Read the model definition and answer for the solid it produces. Units are mm, in the model's axes. Coordinates: 2 decimals unless noted, no trailing zeros. Order: outer loops, then holes, each group sorted by start corner. A loop starts at its lowest first (then second) coordinate and runs counter-clockwise, first axis right, second up. Notation, with made-up numbers: M 36.25,39.5 L 87.25,39.5 A29 cw 87.25,60.5 Z; hole C -4.75,-5.5 d4. An arc over 180 degrees is marked long. Use a Markdown table: item, result. Add a question column.
1) Find section C-C on y = -21.5. Write down the section's boundary in (x, z), plus the area to 3 significant figures.
2) Find section A-A on z = 1.6. Write down the section's boundary in (x, y).
3) Find the intervals of material crossed by probe 1 along Y at (x, z) = (126.5, 1.55); probe 2 along Y at (x, z) = (124.5, 1.7); probe 3 along X at (y, z) = (5.5, 0.7), in increasing order. Write a range as [from, to].
4) The mould has two halves that part along X. Classify faces 1 (the face through (159.386, 1.553, 1.972)), 2 (the face through (18, -14, 0)), 3 (the face through (-62.32, -15.34, 1.97)), 4 (the face through (139.64, -15, 1.97)): released by +X, released by -X, zero draft, split by the parting line, or undercut.
5) Find section B-B on x = 15.5. Write down the section's boundary in (y, z), plus the area to 3 significant figures.
from build123d import *

# Parameters (mm, degrees)
BOSS_EXTRUDE1_DEPTH = 4
FILLET1_R           = 2
FILLET2_R           = 6


with BuildPart() as part:
    # Sketch1 → Boss-Extrude1 (new body)
    with BuildSketch(Plane.XY):
        Polygon((0, 0), (145, 0), (148.090169944, -9.510565163), (157.125206849, -6.574903716), (152.040911292, 9.072949017), (154.894080841, 10), (166.551226371, -11.92390211), (147.252212567, -18.194531813), (132.5, -12), (0, -26.511110048), (-119.286760587, -39.57513503), (-122.91114097, -30.255056337), align=None)
    extrude(amount=BOSS_EXTRUDE1_DEPTH)

    # Fillet1
    # the kernel refuses this fillet: 2 mm, written as the material it adds along each edge
    with BuildSketch(Plane(origin=(157.125206849, -6.574903716, 0), x_dir=(-0.3090169943749429, 0.951056516295155, 0), z_dir=(0, 0, 1))) as fillet1_piece_1:
        with BuildLine():
            CenterArc((FILLET1_R, FILLET1_R), FILLET1_R, 180, 90)
            Line((0, FILLET1_R), (0, 0))
            Line((0, 0), (FILLET1_R, 0))
        make_face()
    extrude(amount=4)
    # the kernel refuses this fillet: 2 mm, written as the material it takes off along each edge
    with BuildSketch(Plane(origin=(152.040911292, 9.072949017, -5), x_dir=(0.3090169943749437, -0.9510565162951549, 0), z_dir=(0, 0, 1))) as fillet1_2_piece_1:
        with BuildLine():
            CenterArc((FILLET1_R, FILLET1_R), FILLET1_R, 180, 90)
            Line((0, FILLET1_R), (0, 0))
            Line((0, 0), (FILLET1_R, 0))
        make_face()
    extrude(amount=14, mode=Mode.SUBTRACT)
    with BuildSketch(Plane(origin=(154.894080841, 10, -4.195498156), x_dir=(-0.9510565162951539, -0.3090169943749466, 0), z_dir=(0, 0, 1))) as fillet1_2_piece_2:
        with BuildLine():
            CenterArc((FILLET1_R * 0.839099631177, FILLET1_R), FILLET1_R, 190, 80)
            Line((-FILLET1_R * 0.145708121835, FILLET1_R * 0.826351822333), (0, 0))
            Line((0, 0), (FILLET1_R * 0.839099631177, 0))
        make_face()
    extrude(amount=12.390996312, mode=Mode.SUBTRACT)

    # Fillet2
    fillet2_edges = [part.edges().sort_by_distance(p)[0] for p in [
        (166.551226371, -11.92390211, 2),
        (147.252212567, -18.194531813, 2),
        (132.5, -12, 2),
    ]]
    fillet(fillet2_edges, radius=FILLET2_R)


solid = part.part
Check result:
| question | item | result |
|---|---|---|
| 1 | outline | M -87.34,0 L 45.76,0 L 45.76,4 L -87.34,4 Z |
| 1 | area | 532 mm2 |
| 2 | outline | M -122.91,-30.26 L -119.29,-39.58 L 130.96,-12.17 A6 cw 133.93,-12.6 L 145.2,-17.33 A6 ccw 149.37,-17.51 L 159.75,-14.13 A6 ccw 163.19,-5.61 L 155.68,8.52 A2 ccw 153.63,9.56 A2 ccw 152.66,7.17 L 156.51,-4.67 A2 cw 155.22,-7.19 L 148.09,-9.51 L 145,0 L 0,0 Z |
| 3 | probe 1 | y = [-12.66, 0] |
| 3 | probe 2 | y = [-12.88, 0] |
| 3 | probe 3 | x = [153.2, 157.29] |
| 4 | face 1 | released by +X |
| 4 | face 2 | zero draft |
| 4 | face 3 | released by -X |
| 4 | face 4 | undercut |
| 5 | outline | M -24.81,0 L 0,0 L 0,4 L -24.81,4 Z |
| 5 | area | 99.3 mm2 |
